Geometry: final body of the model. Coordinates: model frame, mm. Face numbers are marked on the shaded views. Coordinates: 2 decimals unless noted, no trailing zeros. Write each loop counter-clockwise with the first axis right and the second up, starting at its lowest first coordinate (ties: lowest second). Pieces come first, ordered by that corner, then holes. Notation, with made-up numbers: (-39, 48) -> (-1, 48) arc R11 cw to (-1, 68) -> close; hole circle Ø4 at (-31, -20). An arc over 180 degrees is marked (long way). One line per item, written item: value.
```python
from build123d import *

# Parameters (mm, degrees)
SKETCH_1_R               = 8.5
EXTRUDE_1_DEPTH          = 150
SKETCH_2_W               = 9.66465271
SKETCH_2_H               = 17.929973808
EXTRUDE_2_DEPTH          = 20
SKETCH_3_R               = 8.930825741
EXTRUDE_3_DEPTH          = 9.7
SKETCH_4_R               = 6.125222913
CUT_EXTRUDE_1_DEPTH      = 9.7
CUT_EXTRUDE_2_DEPTH      = 180.35679912
CUT_EXTRUDE_2_DEPTH_BACK = 180.35679912
SKETCH_5_R               = 18.5
SKETCH_5_R_2             = 8.5
SKETCH_10_R              = 12.560047034
EXTRUDE_5_DEPTH          = 10
SKETCH_11_R              = 7.5
SKETCH_11_R_2            = 1
EXTRUDE_6_DEPTH          = 1
SKETCH_12_R              = 7.5
EXTRUDE_7_DEPTH          = 5
EXTRUDE_8_DEPTH          = 2
EXTRUDE_8_DEPTH_BACK     = 1
SKETCH_13_W              = 5.120094068
SKETCH_13_H              = 5
SKETCH_14_R              = 1
EXTRUDE_9_DEPTH          = 3
SKETCH_15_R              = 1.806178817
SKETCH_15_R_2            = 1.706178817
CUT_EXTRUDE_3_DEPTH      = 0.2
SKETCH_16_R              = 6
CUT_EXTRUDE_2_2_DEPTH    = 130.2


with BuildPart() as part:
    # 草圖1 → 填料-伸長1 (new body)
    with BuildSketch(Plane(origin=(0, 0, 0), x_dir=(1, 0, 0), z_dir=(0, 1, 0))):
        with Locations(Location((0, 0, 0), (0, 0, 270))):
            Circle(SKETCH_1_R)
    extrude(amount=EXTRUDE_1_DEPTH)

    # 草圖2 → 填料-伸長2 (add)
    with BuildSketch(Plane(origin=(0, 150, 0), x_dir=(1, 0, 0), z_dir=(0, 1, 0))):
        Rectangle(SKETCH_2_W, SKETCH_2_H)
    extrude(amount=EXTRUDE_2_DEPTH)

    # 草圖3 → 填料-伸長3 (add)
    with BuildSketch(Plane(origin=(4.832326355, 0, 0), x_dir=(0, 0, -1), z_dir=(1, 0, 0))):
        with Locations((0, 170)):
            Circle(SKETCH_3_R)
    extrude(amount=-EXTRUDE_3_DEPTH)

    # 草圖4 → 除料-伸長1 (cut)
    with BuildSketch(Plane(origin=(4.832326355, 0, 0), x_dir=(0, 0, -1), z_dir=(1, 0, 0))):
        with Locations((0, 170)):
            Circle(SKETCH_4_R)
    extrude(amount=-CUT_EXTRUDE_1_DEPTH, mode=Mode.SUBTRACT)

    # 草圖5 → Cut-Extrude 2 (cut, two sides: drawn at the far end of the back side and taken through both)
    with BuildSketch(Plane.XZ.offset(-CUT_EXTRUDE_2_DEPTH_BACK)):
        Circle(SKETCH_5_R)
        Circle(SKETCH_5_R_2, mode=Mode.SUBTRACT)
    extrude(amount=CUT_EXTRUDE_2_DEPTH + CUT_EXTRUDE_2_DEPTH_BACK, mode=Mode.SUBTRACT)

    # 草圖9 → 旋轉3 (revolve)
    with BuildSketch(Plane(origin=(0, 0, 0), x_dir=(0, 0, -1), z_dir=(1, 0, 0)), mode=Mode.PRIVATE) as revolve_3_sk:
        Polygon((0, 0), (-9.863847944, 0), (-12.560047034, -4.59966966), (0, -4.59966966), align=None)
    revolve(revolve_3_sk.sketch.rotate(Axis((0, -4.59966966, 0), (0, 1, 0)), 180), axis=Axis((0, -4.59966966, 0), (0, 1, 0)))

    # 草圖10 → 填料-伸長5 (add)
    with BuildSketch(Plane.XZ.offset(4.59966966)):
        with Locations(Location((0, 0, 0), (0, 0, 270))):
            Circle(SKETCH_10_R)
    extrude(amount=EXTRUDE_5_DEPTH)

    # 草圖11 → 填料-伸長6 (add)
    with BuildSketch(Plane.XZ.offset(14.59966966)):
        with Locations(Location((0, 0, 0), (0, 0, 270))):
            Circle(SKETCH_11_R)
        with Locations(Location((-7.188213253, 7.761132083, 0), (0, 0, 270))):
            Circle(SKETCH_11_R_2)
        with Locations(Location((-9.69284226, 4.320867156, 0), (0, 0, 270))):
            Circle(SKETCH_11_R_2)
        with Locations(Location((6.750188429, 7.761132083, 0), (0, 0, 270))):
            Circle(SKETCH_11_R_2)
        with Locations(Location((9.740976841, 4.320867156, 0), (0, 0, 270))):
            Circle(SKETCH_11_R_2)
        with Locations(Location((-3.170732664, -10.604081457, 0), (0, 0, 270))):
            Circle(SKETCH_11_R_2)
        with Locations(Location((2.605242012, -10.604081457, 0), (0, 0, 270))):
            Circle(SKETCH_11_R_2)
    extrude(amount=EXTRUDE_6_DEPTH)

    # 草圖12 → 填料-伸長7 (add)
    with BuildSketch(Plane.XZ.offset(15.59966966)):
        with Locations(Location((0, 0, 0), (0, 0, 270))):
            Circle(SKETCH_12_R)
    extrude(amount=EXTRUDE_7_DEPTH)

    # 草圖13 → 填料-伸長8 (add, two sides: drawn at the far end of the back side and taken through both)
    with BuildSketch(Plane.XY.offset(13).offset(-EXTRUDE_8_DEPTH_BACK)):
        with Locations((0, -12.09966966)):
            Rectangle(SKETCH_13_W, SKETCH_13_H)
    extrude(amount=EXTRUDE_8_DEPTH + EXTRUDE_8_DEPTH_BACK)

    # 草圖14 → 填料-伸長9 (add)
    with BuildSketch(Plane(origin=(0, -9.59966966, 0), x_dir=(1, 0, 0), z_dir=(0, 1, 0))):
        with Locations(Location((0, -13.8, 0), (0, 0, 270))):
            Circle(SKETCH_14_R)
    extrude(amount=EXTRUDE_9_DEPTH)

    # 草圖15 → 除料-伸長-薄件3 (cut)
    with BuildSketch(Plane.XY.offset(15)):
        with Locations((0, -12.122115246)):
            Circle(SKETCH_15_R)
        with Locations((0, -12.122115246)):
            Circle(SKETCH_15_R_2, mode=Mode.SUBTRACT)
    extrude(amount=-CUT_EXTRUDE_3_DEPTH, mode=Mode.SUBTRACT)

    # 草圖16 → Cut-Extrude 2 2 (cut)
    with BuildSketch(Plane.XZ.offset(20.59966966)):
        with Locations(Location((0, 0, 0), (0, 0, 270))):
            Circle(SKETCH_16_R)
    extrude(amount=-CUT_EXTRUDE_2_2_DEPTH, mode=Mode.SUBTRACT)


solid = part.part
```
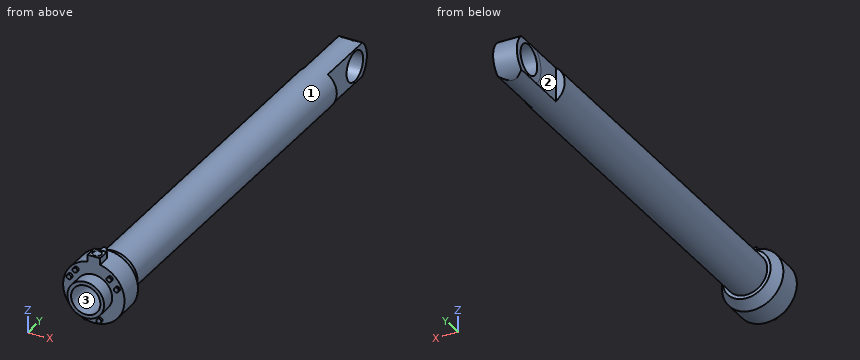
(1) Pull-direction query (Z, two-part tool) for the marked faces 1, 2 and 3; classes: released by +Z, released by -Z, zero draft, split by the parting line, or undercut.
Responses:
face 1: split by the parting line
face 2: zero draft
face 3: undercut
(2) Section A-A (y = 170). Return the cut outline in (x, z), then the cut area to 3 significant figures.
Responses:
outline: (-4.87, -6.97) arc R8.5 ccw to (4.83, -6.99) -> (4.83, -6.13) -> (-4.87, -6.13) -> close; (-4.87, 6.13) -> (4.83, 6.13) -> (4.83, 6.99) arc R8.5 ccw to (-4.87, 6.97) -> close
area: 36.6 mm2
(3) First-contact query: pin 1 (3 mm diameter, centred on x = 6.5, z = -2, fed in from +Y); pin 2 (1.6 mm diameter, centred on x = -3.5, z = -10.5, fed in from -Y); pin 3 (1 mm diameter, centred on x = -6.5, y = 14, fed in from -Z). Flat tips, straight axial feed; report the tip coordinate or a pass-through.
Responses:
pin 1: stops at y = 150
pin 2: stops at y = -15.6
pin 3: stops at z = -6.02
(4) Section B-B (y = 18). Return the cut outline in (x, z).
Responses:
outline: circle Ø17 at (0, 0); hole circle Ø12 at (0, 0)
(5) Line query: line 1 (X direction, y = 65, z = 0); line 2 (Y direction, x = -7.25, z = 7.5); line 3 (Z direction, x = 6, y = 112.5). Output: solid intervals per line, ascending. Write a range as [from, to].
Responses:
line 1: x = [-8.5, -6], [6, 8.5]
line 2: y = [-15.6, -0.97]
line 3: z = [-6.02, 6.02]
